Work out the finished part from the listing and answer in its coordinate system (mm). A direction names the side the tool comes from. Coordinates: 2 decimals unless noted, no trailing zeros. Write each loop counter-clockwise with the first axis right and the second up, starting at its lowest first coordinate (ties: lowest second). Pieces come first, ordered by that corner, then holes. Notation, with made-up numbers: (35.5, 29) - (43.5, 29) arc R31 ccw to (43.5, 58) - close; hole circle Ø4 at (-9.5, 64.25). An arc over 180 degrees is marked (long way). One line per item, written item: value.
Autodesk Inventor part; units mm, degrees
ref_plane "YZ Plane" through (0, 0, 0) normal (1, 0, 0) x (0, 1, 0)
ref_plane "XZ Plane" through (0, 0, 0) normal (0, 1, 0) x (-1, 0, 0)
ref_plane "XY Plane" through (0, 0, 0) normal (0, 0, 1) x (1, 0, 0)
sketch "Sketch1" plane through (0, 0, 0) normal (0, 1, 0) x (-1, 0, 0)
  line L0 (80, 0) -> (80, -250)
  line L1 (80, -250) -> (-80, -250)
  line L2 (-80, -250) -> (-80, 250)
  line L3 (-80, 250) -> (80, 250)
  line L4 (80, 250) -> (80, 0)
  point P0 (0, 0)
extrude "Extrusion1" add sketch "Sketch1" along normal blind 5
sketch "Sketch2" plane through (0, 5, 0) normal (0, 1, 0) x (1, 0, 0)
  line L0 (0, 0) -> (0, -200)
  line L1 (0, -200) -> (10, -200)
  line L2 (10, -200) -> (-10, -200)
  line L3 (-10, -200) -> (-10, -240)
  line L4 (-10, -240) -> (10, -240)
  line L5 (10, -240) -> (10, -200)
  dimension "d7" = 200
  dimension "d8" = 10
  dimension "d9" = 20
  dimension "d10" = 40
  dimension "d11" = 20
extrude "Extrusion2" add sketch "Sketch2" along normal blind 100
sketch "Sketch3" plane through (10, 5, 240) normal (1, 0, 0) x (0, 0, -1)
  line L0 (40, 100) -> (0, 100)
  circle A0 centre (20, 70) radius 7.5
  point P0 (240, -5)
  dimension "d15" = 15
extrude "Extrusion3" cut sketch "Sketch3" against normal blind 100
sketch "Sketch4" plane through (80, 0, 250) normal (1, 0, 0) x (0, 0, -1)
  line L0 (0, 0) -> (0, 5)
  line L1 (0, 0) -> (500, 0)
  line L2 (0, 5) -> (500, 5)
  line L3 (500, 5) -> (500, 0)
  line L4 (500, 0) -> (0, 0)
  line L5 (0, 0) -> (0, 5)
  point P0 (250, 0)
extrude "Extrusion4" add sketch "Sketch4" along normal blind 10
sketch "Sketch5" plane through (-80, 0, -250) normal (-1, 0, 0) x (0, 0, 1)
  line L0 (0, 5) -> (500, 5)
  line L1 (500, 0) -> (500, 5)
  line L2 (0, 5) -> (500, 5)
  line L3 (500, 5) -> (500, 0)
  line L4 (500, 0) -> (0, 0)
  line L5 (0, 0) -> (0, 5)
  point P0 (250, 0)
extrude "Extrusion5" add sketch "Sketch5" along normal blind 10
sketch "Sketch6" plane through (90, 0, -250) normal (0, 0, -1) x (-1, 0, 0)
  line L0 (0, 5) -> (180, 5)
  line L1 (180, 0) -> (0, 0)
  line L2 (0, 5) -> (180, 5)
  line L3 (180, 5) -> (180, 0)
  line L4 (180, 0) -> (0, 0)
  line L5 (0, 0) -> (0, 5)
  point P0 (90, 0)
extrude "Extrusion6" cut sketch "Sketch6" against normal blind 30
sketch "Sketch7" plane through (0, 5, 0) normal (0, 1, 0) x (1, 0, 0)
  line L0 (-90, -250) -> (90, -250)
  arc A0 (79.52, -235.7841) -> (84.52, -235.7841) centre (82.02, -235.7841) ccw
  arc A1 (84.52, 203.719) -> (79.52, 203.719) centre (82.02, 203.719) ccw
  line L1 (79.52, 203.719) -> (79.52, -235.7841)
  line L2 (84.52, -235.7841) -> (84.52, 203.719)
  line L3 (-90, -250) -> (-90, 220)
  line L4 (90, 220) -> (-90, 220)
  arc A2 (-79.52, 203.719) -> (-84.52, 203.719) centre (-82.02, 203.719) ccw
  arc A3 (-84.52, -235.7841) -> (-79.52, -235.7841) centre (-82.02, -235.7841) ccw
  line L5 (-84.52, -235.7841) -> (-84.52, 203.719)
  line L6 (-79.52, 203.719) -> (-79.52, -235.7841)
  point P0 (0, 0)
  dimension "d25" = 5
  dimension "d26" = 5
  dimension "d28" = 5
  dimension "d29" = 5
extrude "Extrusion7" cut sketch "Sketch7" against normal blind 30
sketch "Sketch8" plane through (10, 5, 240) normal (1, 0, 0) x (0, 0, -1)
  point P0 (240, -5)
sketch "Sketch9" plane through (0, 105, 0) normal (0, 1, 0) x (1, 0, 0)
  line L0 (10, -240) -> (-10, -240)
  line L1 (-10, -200) -> (10, -200)
  line L2 (-10, -240) -> (10, -240)
  line L3 (10, -240) -> (10, -200)
  line L4 (10, -200) -> (-10, -200)
  line L5 (-10, -200) -> (-10, -240)
  point P0 (0, 0)
extrude "Extrusion8" cut sketch "Sketch9" against normal blind 16.75
sketch "Sketch10" plane through (-10, 5, 200) normal (-1, 0, 0) x (0, 0, 1)
  line L0 (0, 0) -> (0, 83.25)
  line L1 (40, 0) -> (40, 83.25)
  line L2 (0, 83.25) -> (40, 83.25)
  line L3 (40, 83.25) -> (40, 0)
  line L4 (40, 0) -> (0, 0)
  line L5 (0, 0) -> (0, 83.25)
  circle A0 centre (20, 70) radius 7.5
  circle A1 centre (20, 70) radius 7.5
  point P0 (-200, -5)
extrude "Extrusion9" add sketch "Sketch10" along normal blind 9.5
sketch "Sketch11" plane through (10, 5, 200) normal (0, 0, -1) x (-1, 0, 0)
  line L0 (0, 0) -> (0, 83.25)
  line L1 (0, 0) -> (18.187, 0)
  line L2 (18.187, 0) -> (18.187, 48.2097)
  line L3 (18.187, 48.2097) -> (0, 48.2097)
  line L4 (0, 48.2097) -> (0, 0)
  point P0 (10, -5)
extrude "Extrusion10" cut sketch "Sketch11" against normal blind 66.75
sketch "Sketch12" plane through (10, 88.25, 240) normal (1, 0, 0) x (0, 0, -1)
  line L0 (0, -83.25) -> (0, 0)
  line L1 (40, 0) -> (40, -83.25)
  line L2 (0, -35.059) -> (40, -35.059)
  line L3 (40, -35.059) -> (40, -23.8514)
  line L4 (40, -23.8514) -> (0, -23.8514)
  line L5 (0, -23.8514) -> (0, -35.059)
  point P0 (240, -88.25)
extrude "Extrusion11" cut sketch "Sketch12" against normal blind 18.25
fillet "Fillet1" radius 15 2 edges at (-4.75, 88.25, 240) (-4.75, 88.25, 200)
equation "\"BendRadius\" = Thickness"
equation "\"BendReliefWidth\" = Thickness"
equation "\"BendReliefDepth\" = 0.5 * Thickness"
equation "\"CornerReliefSize\" = 4 * Thickness"
equation "\"MinimumRemnant\" = 2 * Thickness"
equation "\"TransitionRadius\" = BendRadius"
equation "\"JacobiRadiusSize\" = BendRadius"
equation "\"GapSize\" = Thickness"
Item 1: Which of the six approach directions +Z, -Z, +X, -X, +Y, -Y give full straight-line access (tool end or side, diameter ignored) to faces 4 (the face through (-12, 39, 240)), 5 (the face through (10, 81.5, 215.8)), 6 (the face through (-8.25, 59, 220))?
Evaluation:
face 4: +Z, +X, -X, +Y
face 5: +Z, -Z, +X, +Y
face 6: +Z, -Z, +X
Item 2: Consider probe 1 along Y at (x, z) = (1.75, 220); probe 2 along Z at (x, y) = (-10.75, 75); probe 3 along Y at (x, z) = (-11.5, 220). Determine where each line is inside the solid, lowest interval first.
Evaluation:
probe 1: y = 0 to 5, 64.4 to 67.5, 82.5 to 88.25
probe 2: z = 200.1 to 212.5, 227.5 to 239.9
probe 3: y = 0 to 67.5, 82.5 to 88.25
Item 3: Section B-B, the plane z = 220 is taken. Determine the outline of the cut face in (x, y).
Evaluation:
outline: (-90, 0) - (-84.52, 0) - (-84.52, 5) - (-90, 5) - close; (-79.52, 0) - (79.52, 0) - (79.52, 5) - (-8.19, 5) - (-8.19, 53.19) - (-8.25, 53.19) - (-8.25, 64.4) - (10, 64.4) - (10, 67.5) - (-19.5, 67.5) - (-19.5, 5) - (-79.52, 5) - close; (-19.5, 82.5) - (10, 82.5) - (10, 88.25) - (-19.5, 88.25) - close; (84.52, 0) - (90, 0) - (90, 5) - (84.52, 5) - close
Item 4: Section C-C, the plane x = -58.5 is taken. Determine the outline of the cut face in (y, z).
Evaluation:
outline: (0, -220) - (5, -220) - (5, 250) - (0, 250) - close
Item 5: Given pin 1 (19 mm diameter, centred on y = 80.5, z = 219.5, fed in from +X); pin 2 (23.5 mm diameter, centred on x = -11, y = 43.5, fed in from +Z); pin 3 (9 mm diameter, centred on x = 4.5, z = 230, fed in from -Y); pin 4 (23.5 mm diameter, centred on x = 1.5, y = 22.5, fed in from -Z), each flat-ended and moving along its own axis, determine where each tip first touches the part or whether it passes through.
Evaluation:
pin 1: stops at x = 10
pin 2: stops at z = 240
pin 3: stops at y = 0
pin 4: stops at z = 200
Item 6: Determine the mould class of faces 1 (the face through (-11, 46, 200)), 2 (the face through (-4.544, 82.484, 219.506)), 3 (the face through (-4.54, 83.74, 204.28)) for opening direction Y: +Y half, -Y half, draft (parallel to the pull), parting line (faces both ways), or undercut.
Evaluation:
face 1: draft
face 2: undercut
face 3: +Y half
Item 7: Section A-A, the plane z = 3 is taken. Determine the outline of the cut face in (x, y), then the cut area to 3 significant figures.
Evaluation:
outline: (-90, 0) - (-84.52, 0) - (-84.52, 5) - (-90, 5) - close; (-79.52, 0) - (79.52, 0) - (79.52, 5) - (-79.52, 5) - close; (84.52, 0) - (90, 0) - (90, 5) - (84.52, 5) - close
area: 850 mm2
